Job drawing, mm, ordinate dimensions from the low corner. One solid piece. Round coordinates to 2 decimals unless told otherwise and drop trailing zeros. Loops run counter-clockwise (first coordinate to the right, second up) from the corner with the lowest first, then second, coordinate; pieces in that order, holes last.
1) Probe line 1 (X direction, y = 14, z = 0.1); line 2 (Y direction, x = 207, z = 1.6); line 3 (X direction, y = 36, z = 2.3). List the from-to ranges inside material, lowest first.
2) Band-saw the part on A-A, the plane z = 0.55. Write the cut outline in (x, y), then the cut area to 3 significant figures.
3) Drop flat-ended pins along their axis: P1, Ø0.9, axis at y = 45.5, z = 2, coming from the +X side; P2, Ø7, axis at x = 207, y = 14, coming from the +Z side; P3, Ø5.5, axis at x = 389, y = 14, coming from the -Z side; P4, Ø0.9, axis at x = 72.5, z = 1, coming from the +Y side. Give the stop position or say it passes through.
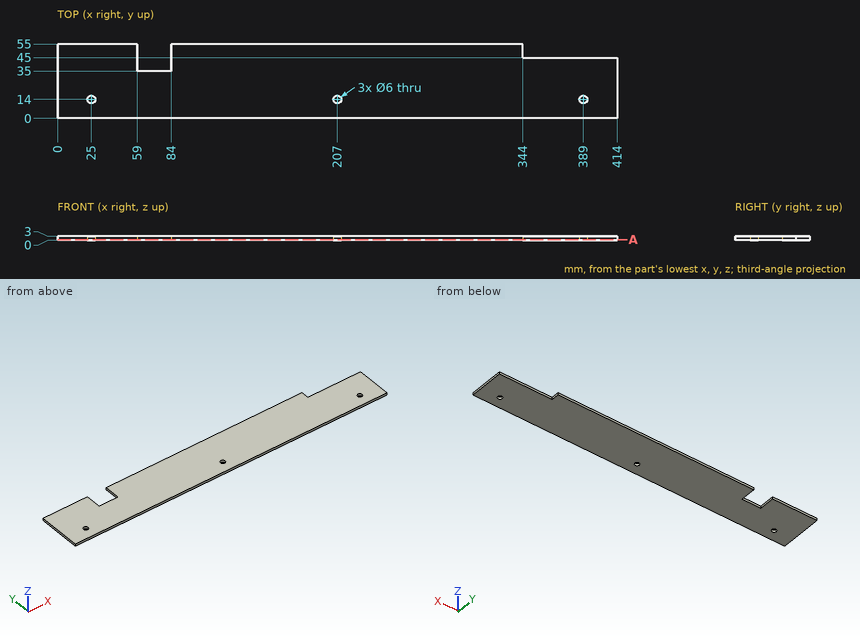
Reported:
1. line 1: x = 0 to 22, 28 to 204, 210 to 386, 392 to 414
1. line 2: y = 0 to 11, 17 to 55
1. line 3: x = 0 to 59, 84 to 414
2. outline: (0, 0) - (414, 0) - (414, 45) - (344, 45) - (344, 55) - (84, 55) - (84, 35) - (59, 35) - (59, 55) - (0, 55) - close; hole circle Ø6 at (25, 14); hole circle Ø6 at (207, 14); hole circle Ø6 at (389, 14)
2. area: 21,500 mm2
3. P1: stops at x = 344
3. P2: stops at z = 3
3. P3: passes through
3. P4: stops at y = 35
